For this review, take the finished solid that the model builds, in its own axes (mm). Face numbers are marked on the shaded views. A direction names the side the tool comes from. Give positions to 0.01 mm unless a question says otherwise; leave off trailing zeros. Order: outer loops, then holes, each group sorted by start corner. A loop starts at its lowest first (then second) coordinate and runs counter-clockwise, first axis right, second up. Notation, with made-up numbers: (11, 44.5) -> (69, 44.5) arc R26 ccw to (69, 82.5) -> close; hole circle Ø8 at (40, 71.5). An arc over 180 degrees is marked (long way). Return JSON: item names as keys, results as strings. Group by question number.
1) Add section A-A (x = 56). Give the boundary of the cut face in (y, z), then the cut area to 3 significant figures.
2) For the marked faces 1 and 2, list the 3-axis set-ups (+Z, -Z, +X, -X, +Y, -Y) from which the entire face can be reached by the end or side of a thin tool; tool diameter is ignored.
3) Insertion check: P1, Ø6, axis at x = -5, y = -3, coming from the +Z side; P2, Ø1, axis at x = 60, y = 6.5, coming from the -Z side; P3, Ø3, axis at x = -6, y = 18, coming from the +Z side; P4, Ø16, axis at x = 0, y = 0, coming from the -Z side. Each pin has a flat end and moves straight along its axis. Give the tip position at first contact, or say it passes through.
4) The part is to be moulded in two halves that separate along Y. For the marked faces 3, 4 and 5, say which applies: released by +Y, released by -Y, zero draft, split by the parting line, or undercut.
5) Add section D-D (z = 36). Give the boundary of the cut face in (x, y).
6) Add section B-B (y = 0). Give the boundary of the cut face in (x, z), then the cut area to 3 significant figures.
7) Add section C-C (x = 0). Give the boundary of the cut face in (y, z).
8) To check wall thickness, follow line 1 along Y through (x, z) = (0, 60); line 2 along X through (y, z) = (0, 28); line 3 along Z through (x, y) = (-23, 21.5). State the ranges of each line that lie inside material, in increasing order.
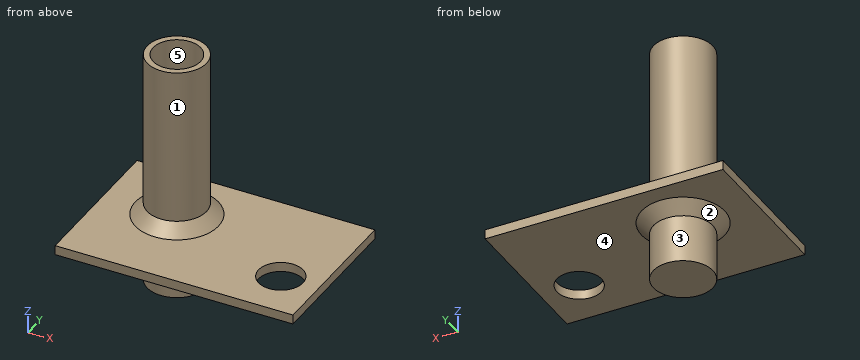
from build123d import *

# Parameters (mm, degrees)
F0_R     = 12.5
F1_DEPTH = 100
F2_T     = -2.5
F4_W     = 100
F4_H     = 65
F4_R     = 9.376015
F4_R_2   = 12.5
F5_DEPTH = 4
F6_SIZE  = 5


with BuildPart() as f1:
    # F0 (on Top) → F1 (new body)
    with BuildSketch(Plane.XY):
        Circle(F0_R)
    extrude(amount=F1_DEPTH)

    # F2
    f2_openings = [f1.faces().sort_by_distance(p)[0] for p in [
        (0, 0, 100),
    ]]
    offset(amount=F2_T, openings=f2_openings)

    # F4 (on offset) → F5 (join)
    with BuildSketch(Plane.XY.offset(25)):
        with Locations((20, -7.5)):
            Rectangle(F4_W, F4_H)
        with Locations((53.792767, -19.060429)):
            Circle(F4_R, mode=Mode.SUBTRACT)
        Circle(F4_R_2, mode=Mode.SUBTRACT)
    extrude(amount=F5_DEPTH)

    # F6
    f6_edges = [f1.edges().sort_by_distance(p)[0] for p in [
        (-12.5, 0, 29),
        (-12.5, 0, 25),
    ]]
    chamfer(f6_edges, length=F6_SIZE)


solid = f1.part
Evaluation:
{
 "1": {"outline": "(-40, 25) -> (-28.17, 25) -> (-28.17, 29) -> (-40, 29) -> close; (-9.95, 25) -> (25, 25) -> (25, 29) -> (-9.95, 29) -> close", "area": "187 mm^2"},
 "2": {"face 1": "+Z", "face 2": "-Z"},
 "3": {"P1": "z = 2.5", "P2": "z = 25", "P3": "z = 29.03", "P4": "z = 0"},
 "4": {"face 3": "split by the parting line", "face 4": "zero draft", "face 5": "undercut"},
 "5": {"outline": "circle Ø25 at (0, 0); hole circle Ø20 at (0, 0)"},
 "6": {"outline": "(-30, 25) -> (-17.5, 25) -> (-12.5, 20) -> (-12.5, 0) -> (12.5, 0) -> (12.5, 20) -> (17.5, 25) -> (70, 25) -> (70, 29) -> (17.5, 29) -> (12.5, 34) -> (12.5, 100) -> (10, 100) -> (10, 2.5) -> (-10, 2.5) -> (-10, 100) -> (-12.5, 100) -> (-12.5, 34) -> (-17.5, 29) -> (-30, 29) -> close", "area": "900 mm^2"},
 "7": {"outline": "(-40, 25) -> (-17.5, 25) -> (-12.5, 20) -> (-12.5, 0) -> (12.5, 0) -> (12.5, 20) -> (17.5, 25) -> (25, 25) -> (25, 29) -> (17.5, 29) -> (12.5, 34) -> (12.5, 100) -> (10, 100) -> (10, 2.5) -> (-10, 2.5) -> (-10, 100) -> (-12.5, 100) -> (-12.5, 34) -> (-17.5, 29) -> (-40, 29) -> close"},
 "8": {"line 1": "-12.5 to -10, 10 to 12.5", "line 2": "-30 to -10, 10 to 70", "line 3": "25 to 29"}
}
